Here's the drawing with two shaded views (mm, measured from the low corner). I have some questions. Give positions to 0.01 mm unless a question says otherwise; leave off trailing zeros. Loops run counter-clockwise (first coordinate to the right, second up) from the corner with the lowest first, then second, coordinate; pieces in that order, holes last. Notation, with made-up numbers: (44, 48.5) - (102, 48.5) arc R30 cw to (102, 80.5) - close; hole circle Ø3 at (26.25, 23.25). An arc over 180 degrees is marked (long way). Answer as a JSON object with one key per item and string values. Group by question number.
Item 1: Suppose I cut it at D-D on x = 162. Write out the boundary of the cut face in (y, z), and give its area (3 significant figures).
Item 2: Please list where these lines run through material, in increasing order: L1, parallel to Z at x = 200, y = 57; L2, parallel to Z at x = 127, y = 57; L3, parallel to Z at x = 111, y = 65.
Item 3: Suppose I cut it at C-C on z = 87. Write out the boundary of the cut face in (x, y), and give its area (3 significant figures).
Item 4: Suppose I cut it at A-A on y = 100. Write out the boundary of the cut face in (x, z) (1 decimal).
Item 5: Thinking about a two-plate mould opening in Z: for the marked faces 1, 2 and 3, which applies, pulls with the +Z half, pulls with the -Z half, needs draft (parallel to the pull), parting line crosses it, or undercut?
Item 6: Suppose I cut it at B-B on y = 57. Count the separate pieces of the cut face and the enclosed holes in it, and give its area (3 significant figures).
Item 7: Will these pins go through, and if not, where does the flat tip stop? pin 1 (6.5 mm diameter, centred on x = 300, z = 143.25, fed in from -Y); pin 2 (11 mm diameter, centred on x = 253.5, z = 140, fed in from +Y); pin 3 (2 mm diameter, centred on x = 215, y = 15.5, fed in from -Z); pin 4 (8 mm diameter, centred on x = 128.5, y = 67, fed in from -Z).
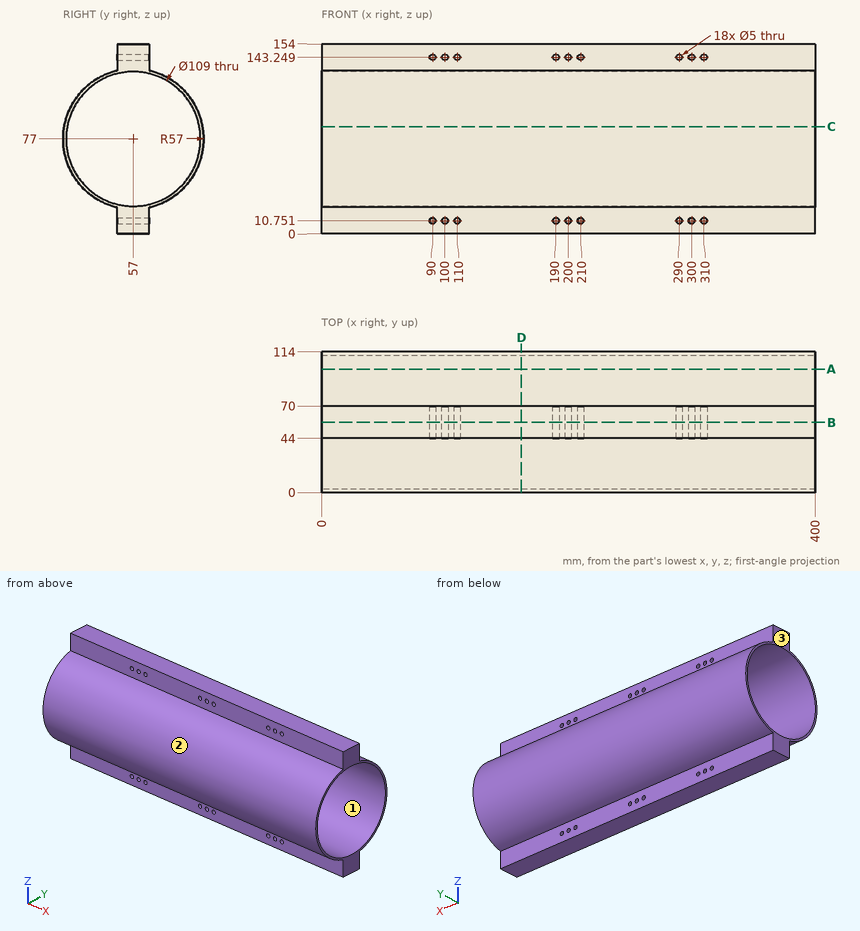
Worked out:
{
 "1": {"outline": "(44, 0) - (70, 0) - (70, 21.5) arc R57 ccw to (70, 132.5) - (70, 154) - (44, 154) - (44, 132.5) arc R57 ccw to (44, 21.5) - close; hole circle Ø109 at (57, 77)", "area": "1,940 mm2"},
 "2": {"L1": "z = 0 to 8.25, 13.25 to 22.5, 131.5 to 140.75, 145.75 to 154", "L2": "z = 0 to 22.5, 131.5 to 154", "L3": "z = 0 to 8.46, 13.04 to 23.09, 130.91 to 140.96, 145.54 to 154"},
 "3": {"outline": "(0, 0.88) - (400, 0.88) - (400, 3.43) - (0, 3.43) - close; (0, 110.57) - (400, 110.57) - (400, 113.12) - (0, 113.12) - close", "area": "2,030 mm2"},
 "4": {"outline": "(0, 39.6) - (400, 39.6) - (400, 43.5) - (0, 43.5) - close; (0, 110.5) - (400, 110.5) - (400, 114.4) - (0, 114.4) - close"},
 "5": {"face 1": "undercut", "face 2": "parting line crosses it", "face 3": "needs draft"},
 "6": {"separate pieces": "2", "enclosed holes": "18", "area": "17,600 mm2"},
 "7": {"pin 1": "stops at y = 44", "pin 2": "stops at y = 70", "pin 3": "stops at z = 36.89", "pin 4": "stops at z = 0"}
}
